Check sheet for the modelled part. Datum: model origin and axes. Units: mm. A direction names the side the tool comes from. Give positions to 0.01 mm unless a question says otherwise; leave off trailing zeros. Write each loop counter-clockwise with the first axis right and the second up, starting at its lowest first coordinate (ties: lowest second). Pieces come first, ordered by that corner, then holes. Notation, with made-up numbers: M -2,38 L 11,38 A19 ccw 11,75 Z; hole C 66,12 d1. An arc over 180 degrees is marked long. Use CSV: the item, a comma, the result in double quotes. Start each with the question number.
1. Cross-section at A-A, the plane y = -0.55. Enter the section's corners in (x, z), and give its area (3 significant figures).
2. Access from +Z, -Z, +X, -X, +Y, -Y to the whole of each face (thin tool, end or side, straight path). Record for faces 1 (the face through (-1.293, 0.761, -12.675)), 2 (the face through (-0.63, -1.073, -29.275)), 3 (the face through (-1.305, -0.739, -12.675)).
3. Depth check by flat-ended pin: P1, Ø2, axis at x = -1.5, z = -15.5, coming from the -Y side; P2, Ø1.5, axis at y = -1, z = -24, coming from the -X side. Enter the tip coordinate at first touch or a pass-through.
4. Cross-section at D-D, the plane y = 0.95. Enter the section's corners in (x, z).
5. Cross-section at C-C, the plane z = -12. Enter the section's corners in (x, y).
6. Cross-section at B-B, the plane x = -8.75. Enter the section's corners in (y, z), and give its area (3 significant figures).
7. Scan lines: line 1 (Z direction, x = -6.75, y = -0.75); line 2 (Z direction, x = -6.5, y = 0.15); line 3 (X direction, y = 1.35, z = -22). Record each from-to range of solid material in increasing order.
Autodesk Inventor part; units mm, degrees
ref_plane "YZ Plane" through (0, 0, 0) normal (1, 0, 0) x (0, 1, 0)
ref_plane "XZ Plane" through (0, 0, 0) normal (0, 1, 0) x (-1, 0, 0)
ref_plane "XY Plane" through (0, 0, 0) normal (0, 0, 1) x (1, 0, 0)
sketch "Esquisse1" plane through (0, 0, 0) normal (0, 0, 1) x (1, 0, 0)
  line L0 (0.866, -1.5) -> (-0.866, -1.5)
  line L1 (-0.866, -1.5) -> (-1.7321, 0)
  line L2 (-1.7321, 0) -> (-0.866, 1.5)
  line L3 (-0.866, 1.5) -> (0.866, 1.5)
  line L4 (0.866, 1.5) -> (1.7321, 0)
  line L5 (1.7321, 0) -> (0.866, -1.5)
  point P0 (0, 0)
  point P1 (0, 0)
  dimension "Taille" = 3
sketch "Esquisse2" plane through (0, 0, 0) normal (0, 1, 0) x (-1, 0, 0)
  line L0 (0, 0) -> (0, -25)
  line L1 (5, -30) -> (10, -30)
  arc A0 (0, -25) -> (5, -30) centre (5, -25) ccw
  point P0 (0, -30)
  dimension "Grand_longueur" = 30
  dimension "Petites_longueur" = 10
  dimension "COngé" = 5
sweep "Balayage1" add profiles "Esquisse1" path "Esquisse2"
properties part number "1420-12 Cle btr-04" material "Acier inoxydable"
Worked answers:
1,outline,"M -10,-31.41 L -5,-31.41 A6.41 ccw 1.41,-25 L 1.41,0 L -1.41,0 L -1.41,-25 A3.59 cw -5,-28.59 L -10,-28.59 Z"
1,area,"107 mm^2"
2,face 1,"+Z, -X, +Y"
2,face 2,"-Z, +X, -Y"
2,face 3,"+Z, -X, -Y"
3,P1,"stops at y = -1.5"
3,P2,"stops at x = -1.59"
4,outline,"M -10,-31.18 L -5,-31.18 A6.18 ccw 1.18,-25 L 1.18,0 L -1.18,0 L -1.18,-25 A3.82 cw -5,-28.82 L -10,-28.82 Z"
5,outline,"M -1.73,0 L -0.87,-1.5 L 0.87,-1.5 L 1.73,0 L 0.87,1.5 L -0.87,1.5 Z"
6,outline,"M -1.5,-30.87 L 0,-31.73 L 1.5,-30.87 L 1.5,-29.13 L 0,-28.27 L -1.5,-29.13 Z"
6,area,"7.79 mm^2"
7,line 1,"z = -31.3 to -28.7"
7,line 2,"z = -31.65 to -28.35"
7,line 3,"x = -0.95 to 0.95"
